from build123d import *

# Parameters (mm, degrees)
SKETCH1_W           = 68
SKETCH1_H           = 33
BOSS_EXTRUDE1_DEPTH = 3.175
FILLET1_R           = 1
SKETCH2_R           = 2.15
SKETCH2_R_2         = 1.7
CUT_EXTRUDE2_DEPTH  = 1.25


with BuildPart() as part:
    # Sketch1 → Boss-Extrude1 (new body)
    with BuildSketch(Plane.XY):
        Rectangle(SKETCH1_W, SKETCH1_H)
    extrude(amount=BOSS_EXTRUDE1_DEPTH)

    # Fillet1
    fillet1_edges = [part.edges().sort_by_distance(p)[0] for p in [
        (34, 16.5, 1.5875),
        (34, -16.5, 1.5875),
        (-34, -16.5, 1.5875),
        (-34, 16.5, 1.5875),
    ]]
    fillet(fillet1_edges, radius=FILLET1_R)

    # Sketch2 → Cut-Extrude2 (cut)
    with BuildSketch(Plane(origin=(0, 0, 0), x_dir=(-1, 0, 0), z_dir=(0, 0, -1))):
        with Locations((20.5, 0)):
            Circle(SKETCH2_R)
        with Locations((31.75, -14.25)):
            Circle(SKETCH2_R_2)
        with Locations(Location((31.75, 14.25, 0), (0, 0, 180))):
            Circle(SKETCH2_R_2)
        with BuildLine():
            Line((-31.75, 15.95), (-29.25, 15.95))
            ThreePointArc((-29.25, 15.95), (-27.55, 14.25), (-29.25, 12.55))
            Line((-29.25, 12.55), (-31.75, 12.55))
            ThreePointArc((-31.75, 12.55), (-33.45, 14.25), (-31.75, 15.95))
        make_face()
        with BuildLine():
            Line((-31.75, -15.95), (-29.25, -15.95))
            ThreePointArc((-29.25, -15.95), (-27.55, -14.25), (-29.25, -12.55))
            Line((-29.25, -12.55), (-31.75, -12.55))
            ThreePointArc((-31.75, -12.55), (-33.45, -14.25), (-31.75, -15.95))
        make_face()
        with BuildLine():
            Line((-20.5, 2.15), (-17.5, 2.15))
            ThreePointArc((-17.5, 2.15), (-15.35, 0), (-17.5, -2.15))
            Line((-17.5, -2.15), (-20.5, -2.15))
            ThreePointArc((-20.5, -2.15), (-22.65, 0), (-20.5, 2.15))
        make_face()
    extrude(amount=-CUT_EXTRUDE2_DEPTH, mode=Mode.SUBTRACT)


solid = part.part
Part model, mm, in its own coordinate system. A direction names the side the tool comes from. Give positions to 0.01 mm unless a question says otherwise; leave off trailing zeros. Write each loop counter-clockwise with the first axis right and the second up, starting at its lowest first coordinate (ties: lowest second). Pieces come first, ordered by that corner, then holes.
1) Cut at C-C on y = 14.25. Write the cut outline in (x, z) (3 decimals).
Resolved:
outline: (-34, 0) - (-33.45, 0) - (-33.45, 1.25) - (-30.05, 1.25) - (-30.05, 0) - (27.55, 0) - (27.55, 1.25) - (33.45, 1.25) - (33.45, 0) - (34, 0) - (34, 3.175) - (-34, 3.175) - close
2) Cut at D-D on x = -31.75. Write the cut outline in (y, z) (3 decimals), then the cut area to 3 significant figures.
Resolved:
outline: (-16.5, 0) - (-15.95, 0) - (-15.95, 1.25) - (-12.55, 1.25) - (-12.55, 0) - (12.55, 0) - (12.55, 1.25) - (15.95, 1.25) - (15.95, 0) - (16.5, 0) - (16.5, 3.175) - (-16.5, 3.175) - close
area: 96.3 mm2
3) Cut at A-A on x = -20.5. Write the cut outline in (y, z) (3 decimals).
Resolved:
outline: (-16.5, 0) - (-2.15, 0) - (-2.15, 1.25) - (2.15, 1.25) - (2.15, 0) - (16.5, 0) - (16.5, 3.175) - (-16.5, 3.175) - close
4) Which spindle directions (+Z, -Z, +X, -X, +Y, -Y) get a long thin tool onto all of the face, cutting with end or side? Do faces 4 (the face through (-34, 0, 2)), 5 (the face through (27.55, 14.29, 0.62)). Say none if no direction does.
Resolved:
face 4: +Z, -Z, -X, +Y, -Y
face 5: -Z
5) Two-plate mould, pull along X, no slides. Class faces 1 (the face through (0, -16.5, 2)), 2 (the face through (34, 0, 2)), 3 (the face through (31, -14, 1.25)): released by +X, released by -X, zero draft, split by the parting line, or undercut.
Resolved:
face 1: zero draft
face 2: released by +X
face 3: undercut
6) Cut at B-B on z = 0.75. Write the cut outline in (x, y), then the cut area to 3 significant figures.
Resolved:
outline: (-34, -15.5) arc R1 ccw to (-33, -16.5) - (33, -16.5) arc R1 ccw to (34, -15.5) - (34, 15.5) arc R1 ccw to (33, 16.5) - (-33, 16.5) arc R1 ccw to (-34, 15.5) - close; hole circle Ø3.4 at (-31.75, -14.25); hole circle Ø3.4 at (-31.75, 14.25); hole circle Ø4.3 at (-20.5, 0); hole (17.5, -2.15) - (20.5, -2.15) arc R2.15 ccw to (20.5, 2.15) - (17.5, 2.15) arc R2.15 ccw to start; hole (29.25, -15.95) - (31.75, -15.95) arc R1.7 ccw to (31.75, -12.55) - (29.25, -12.55) arc R1.7 ccw to start; hole (29.25, 12.55) - (31.75, 12.55) arc R1.7 ccw to (31.75, 15.95) - (29.25, 15.95) arc R1.7 ccw to start
area: 2,150 mm2
7) Probe L1, parallel to Y at x = -31.75, z = 0.3; L2, parallel to X at y = 14.25, z = 1.05; L3, parallel to Z at x = 18, y = 2 (3 decimals). List the from-to ranges inside material, lowest first.
Resolved:
L1: y = -16.5 to -15.95, -12.55 to 12.55, 15.95 to 16.5
L2: x = -34 to -33.45, -30.05 to 27.55, 33.45 to 34
L3: z = 1.25 to 3.175
8) Pin check, flat tip, straight feed: pin 1 (1 mm diameter, centred on x = -32.5, y = -14, fed in from -Z). Stop position of the tip, or through.
Resolved:
pin 1: stops at z = 1.25
